Answer from the drawing. Dimensions are ordinates in mm from the lowest x, y and z of the part. A direction names the side the tool comes from. Round coordinates to 2 decimals unless told otherwise and drop trailing zeros. Order: outer loops, then holes, each group sorted by start corner. A loop starts at its lowest first (then second) coordinate and runs counter-clockwise, first axis right, second up.
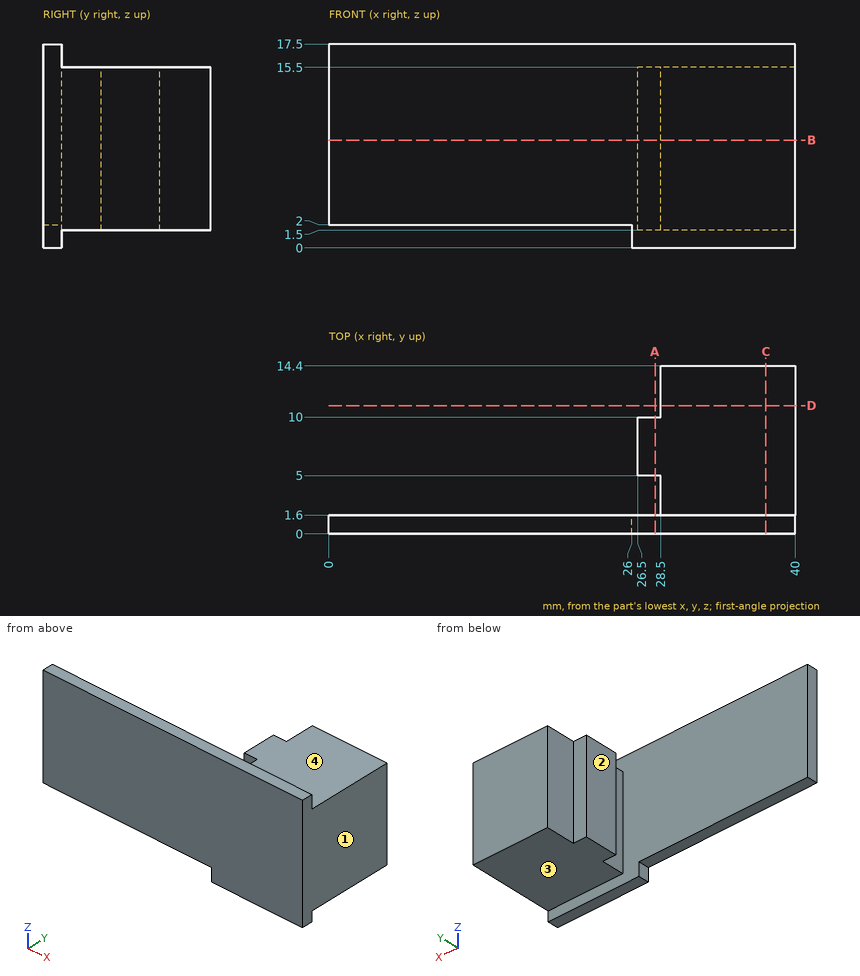
Q1. A cutting plane is placed at B-B, the plane z = 9.25. Give the vertices of the cut face in (x, y).
Outcome:
outline: (0, 0) - (40, 0) - (40, 14.4) - (28.5, 14.4) - (28.5, 10) - (26.5, 10) - (26.5, 5) - (28.5, 5) - (28.5, 1.6) - (0, 1.6) - close
Q2. Straight lines are drawn through the part: probe 1 along Y at (x, z) = (8, 8); probe 2 along Z at (x, y) = (34, 3); probe 3 along X at (y, z) = (3.25, 15). For each, find the intervals that lie inside material, in ascending order.
Outcome:
probe 1: y = 0 to 1.6
probe 2: z = 1.5 to 15.5
probe 3: x = 28.5 to 40
Q3. A cutting plane is placed at D-D, the plane y = 11. Give the vertices of the cut face in (x, z), plus the area to 3 significant figures.
Outcome:
outline: (28.5, 1.5) - (40, 1.5) - (40, 15.5) - (28.5, 15.5) - close
area: 161 mm2
Q4. A cutting plane is placed at C-C, the plane x = 37.5. Give the vertices of the cut face in (y, z), plus the area to 3 significant figures.
Outcome:
outline: (0, 0) - (1.6, 0) - (1.6, 1.5) - (14.4, 1.5) - (14.4, 15.5) - (1.6, 15.5) - (1.6, 17.5) - (0, 17.5) - close
area: 207 mm2
Q5. A cutting plane is placed at A-A, the plane x = 28. Give the vertices of the cut face in (y, z).
Outcome:
outline: (0, 0) - (1.6, 0) - (1.6, 17.5) - (0, 17.5) - close; (5, 1.5) - (10, 1.5) - (10, 15.5) - (5, 15.5) - close
Q6. For the marked faces 1, 2, 3 and 4, determine the directions among +Z, -Z, +X, -X, +Y, -Y from which every point of the face is accessible in a straight line to the end or side of a thin tool.
Outcome:
face 1: +Z, -Z, +X, +Y, -Y
face 2: +Z, -Z, -X, +Y
face 3: -Z, +X, -X, +Y
face 4: +Z, +X, -X, +Y
Q7. Flat-ended cylindrical pins translate along their axes: pin 1 (1.8 mm diameter, centred on x = 9, y = 0.5, fed in from -Z); pin 2 (4 mm diameter, centred on x = 32.5, y = 7.5, fed in from -Z); pin 3 (1.7 mm diameter, centred on y = 3, z = 7, fed in from -X). Find the tip coordinate at first contact, or state that the pin passes through.
Outcome:
pin 1: stops at z = 2
pin 2: stops at z = 1.5
pin 3: stops at x = 28.5
